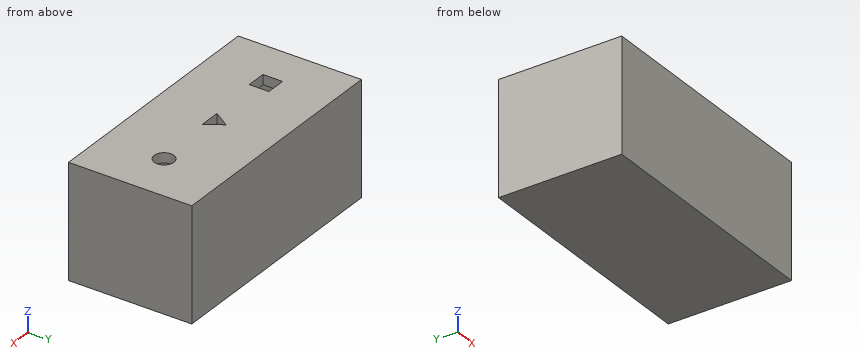
from build123d import *

# Parameters (mm, degrees)
SKETCH1_W           = 250
SKETCH1_H           = 125
SKETCH1_W_2         = 230
SKETCH1_H_2         = 115
BOSS_EXTRUDE1_DEPTH = 100
SKETCH2_W           = 250
SKETCH2_H           = 125
BOSS_EXTRUDE2_DEPTH = 5
SKETCH3_W           = 250
SKETCH3_H           = 125
SKETCH3_W_2         = 230
SKETCH3_H_2         = 115
SKETCH3_R           = 10
SKETCH3_W_3         = 20
SKETCH3_H_3         = 20
BOSS_EXTRUDE4_DEPTH = 10


with BuildPart() as part:
    # Sketch1 → Boss-Extrude1 (new body)
    with BuildSketch(Plane.XY):
        Rectangle(SKETCH1_W, SKETCH1_H)
        Rectangle(SKETCH1_W_2, SKETCH1_H_2, mode=Mode.SUBTRACT)
    extrude(amount=BOSS_EXTRUDE1_DEPTH)

    # Sketch2 → Boss-Extrude2 (add)
    with BuildSketch(Plane(origin=(0, 0, 0), x_dir=(-1, 0, 0), z_dir=(0, 0, -1))):
        Rectangle(SKETCH2_W, SKETCH2_H)
    extrude(amount=BOSS_EXTRUDE2_DEPTH)

    # Sketch3 → Boss-Extrude4 (add)
    # profile 1 of 2: a face of its own
    with BuildSketch(Plane.XY.offset(100)):
        Rectangle(SKETCH3_W, SKETCH3_H)
        Rectangle(SKETCH3_W_2, SKETCH3_H_2, mode=Mode.SUBTRACT)
    # profile 2 of 2: a face of its own
    with BuildSketch(Plane.XY.offset(100)):
        Rectangle(SKETCH3_W_2, SKETCH3_H_2)
        with Locations((75, 0)):
            Circle(SKETCH3_R, mode=Mode.SUBTRACT)
        with Locations((-75, 0)):
            Rectangle(SKETCH3_W_3, SKETCH3_H_3, mode=Mode.SUBTRACT)
        Polygon((0, 11.153858408), (10.958136059, -5.576929204), (-10.958136059, -5.576929204), align=None, mode=Mode.SUBTRACT)
    extrude(amount=BOSS_EXTRUDE4_DEPTH)


solid = part.part
CAD build for the part. Positions are in the model's coordinates, mm. Coordinates: 2 decimals unless noted, no trailing zeros. Order: outer loops, then holes, each group sorted by start corner. A loop starts at its lowest first (then second) coordinate and runs counter-clockwise, first axis right, second up.
Item 1: Pin check, flat tip, straight feed: pin 1 Ø16 at (x, y) = (75, 0) entering from +Z. Stop position of the tip, or through.
Check sheet entries:
pin 1: stops at z = 0
Item 2: Band-saw the part on B-B on y = 0. List the corners of the cut face in (x, z).
Check sheet entries:
outline: (-125, -5) - (125, -5) - (125, 110) - (85, 110) - (85, 100) - (115, 100) - (115, 0) - (-115, 0) - (-115, 100) - (-85, 100) - (-85, 110) - (-125, 110) - close; (-65, 100) - (-7.31, 100) - (-7.31, 110) - (-65, 110) - close; (7.31, 100) - (65, 100) - (65, 110) - (7.31, 110) - close
Item 3: Band-saw the part on D-D on x = 75. List the corners of the cut face in (y, z).
Check sheet entries:
outline: (-62.5, -5) - (62.5, -5) - (62.5, 110) - (10, 110) - (10, 100) - (57.5, 100) - (57.5, 0) - (-57.5, 0) - (-57.5, 100) - (-10, 100) - (-10, 110) - (-62.5, 110) - close
Item 4: Drill centre lines: L1, parallel to Y at x = 63, z = 51.5; L2, parallel to X at y = -53, z = 38.5; L3, parallel to Z at x = 92.5, y = -8. Where is each one in solid material? Low to high.
Check sheet entries:
L1: y = -62.5 to -57.5, 57.5 to 62.5
L2: x = -125 to -115, 115 to 125
L3: z = -5 to 0, 100 to 110
Item 5: Band-saw the part on A-A on z = 25. List the corners of the cut face in (x, y), plus the area to 3 significant figures.
Check sheet entries:
outline: (-125, -62.5) - (125, -62.5) - (125, 62.5) - (-125, 62.5) - close; hole (-115, -57.5) - (115, -57.5) - (115, 57.5) - (-115, 57.5) - close
area: 4,800 mm2
Item 6: Band-saw the part on C-C on x = -40. List the corners of the cut face in (y, z).
Check sheet entries:
outline: (-62.5, -5) - (62.5, -5) - (62.5, 110) - (-62.5, 110) - close; hole (-57.5, 0) - (57.5, 0) - (57.5, 100) - (-57.5, 100) - close
